```python
from build123d import *

# Parameters (mm, degrees)
SKETCH1_W           = 12.7
SKETCH1_H           = 12.7
BOSS_EXTRUDE1_DEPTH = 292.1
CUT_EXTRUDE1_DEPTH  = 13.7
CUT_EXTRUDE2_DEPTH  = 13.7
LPATTERN1_COUNT     = 3
LPATTERN1_PITCH     = 95.25


with BuildPart() as part:
    # Sketch1 → Boss-Extrude1 (new body)
    with BuildSketch(Plane(origin=(0, 0, 0), x_dir=(1, 0, 0), z_dir=(0, 1, 0))):
        Rectangle(SKETCH1_W, SKETCH1_H)
    extrude(amount=BOSS_EXTRUDE1_DEPTH)

    # Sketch2 → Cut-Extrude1 (cut, through all)
    with BuildSketch(Plane(origin=(0, 0, -6.35), x_dir=(-1, 0, 0), z_dir=(0, 0, -1))):
        with BuildLine():
            Line((-2.413, 279.4), (-2.413, 203.2))
            ThreePointArc((-2.413, 203.2), (0, 200.787), (2.413, 203.2))
            Line((2.413, 203.2), (2.413, 279.4))
            ThreePointArc((2.413, 279.4), (0, 281.813), (-2.413, 279.4))
        make_face()
    cut_extrude1 = extrude(amount=-CUT_EXTRUDE1_DEPTH, mode=Mode.SUBTRACT)

    # Sketch3 → Cut-Extrude2 (cut, through all)
    with BuildSketch(Plane(origin=(6.35, 0, 0), x_dir=(0, 0, -1), z_dir=(1, 0, 0))):
        with BuildLine():
            Line((-2.413, 279.4), (-2.413, 203.2))
            ThreePointArc((-2.413, 203.2), (0, 200.787), (2.413, 203.2))
            Line((2.413, 203.2), (2.413, 279.4))
            ThreePointArc((2.413, 279.4), (0, 281.813), (-2.413, 279.4))
        make_face()
    cut_extrude2 = extrude(amount=-CUT_EXTRUDE2_DEPTH, mode=Mode.SUBTRACT)

    # LPattern1: Cut-Extrude1, Cut-Extrude2 ×3
    with Locations(*[(0, -i * LPATTERN1_PITCH, 0) for i in range(1, LPATTERN1_COUNT)]):
        add(cut_extrude1, mode=Mode.SUBTRACT)
        add(cut_extrude2, mode=Mode.SUBTRACT)


solid = part.part
```
Model file for the job. Use its own axes, mm. A direction names the side the tool comes from. Coordinates: 2 decimals unless noted, no trailing zeros. Loops run counter-clockwise (first coordinate to the right, second up) from the corner with the lowest first, then second, coordinate; pieces in that order, holes last. Notation, with made-up numbers: (-3.75, 25.25) -> (5.25, 25.25) arc R18 ccw to (5.25, 39.25) -> close; hole circle Ø4 at (80, 88). An arc over 180 degrees is marked (long way). Answer as a JSON object with one key per item and string values.
Q1. Cut at A-A (y = 138.5). List the corners of the cut face in (x, z).
Report:
{"outline": "(-6.35, -6.35) -> (-2.41, -6.35) -> (-2.41, -2.41) -> (-6.35, -2.41) -> close; (-6.35, 2.41) -> (-2.41, 2.41) -> (-2.41, 6.35) -> (-6.35, 6.35) -> close; (2.41, -6.35) -> (6.35, -6.35) -> (6.35, -2.41) -> (2.41, -2.41) -> close; (2.41, 2.41) -> (6.35, 2.41) -> (6.35, 6.35) -> (2.41, 6.35) -> close"}
Q2. 3-axis set-ups, long thin cutter, end or side, ignore diameter. For faces 4 (the cylindrical face through (3.925, 10.288, 0.053)), 5 (the cylindrical face through (0.053, 105.538, 3.836)), 6 (the flat face through (0, 0, 0)): which of +Z, -Z, +X, -X, +Y, -Y reach the whole face in a straight line?
Report:
{"face 4": "+X, -X", "face 5": "+Z, -Z", "face 6": "+Z, -Z, +X, -X, -Y"}
Q3. Flat gauge pin, fed straight in: P1, Ø1, axis at y = 35, z = 0.5, coming from the -X side. Where does the tip first touch, or does it go through?
Report:
{"P1": "passes through"}
Q4. Pull direction Z, two halves, no side cores. Call faces 1 (the flat face through (3, 144, 6.35)), 2 (the cylindrical face through (-0.053, 281.812, 3.836)), 3 (the cylindrical face through (3.925, 186.562, -0.053)): released by +Z, released by -Z, zero draft, split by the parting line, or undercut.
Report:
{"face 1": "released by +Z", "face 2": "zero draft", "face 3": "undercut"}
Q5. Probe probe 1 along X at (y, z) = (262, 5); probe 2 along Y at (x, z) = (0, -4.75). List the from-to ranges inside material, lowest first.
Report:
{"probe 1": "x = -6.35 to -2.41, 2.41 to 6.35", "probe 2": "y = 0 to 10.29, 91.31 to 105.54, 186.56 to 200.79, 281.81 to 292.1"}
